from build123d import *

# Parameters (mm, degrees)
SKETCH_1_W      = 100
SKETCH_1_H      = 52
SKETCH_1_R      = 1.6
EXTRUDE_1_DEPTH = 3
FILLET_1_R      = 2


with BuildPart() as part:
    # 草图1 → 凸台-拉伸1 (new body)
    with BuildSketch(Plane(origin=(0, 0, 0), x_dir=(1, 0, 0), z_dir=(0, 1, 0))):
        Rectangle(SKETCH_1_W, SKETCH_1_H)
        with Locations(Location((-36.5, 17, 0), (0, 0, 270))):
            Circle(SKETCH_1_R, mode=Mode.SUBTRACT)
        with Locations(Location((36.5, 17, 0), (0, 0, 270))):
            Circle(SKETCH_1_R, mode=Mode.SUBTRACT)
        with Locations(Location((36.5, -19, 0), (0, 0, 270))):
            Circle(SKETCH_1_R, mode=Mode.SUBTRACT)
        with Locations(Location((-36.5, -19, 0), (0, 0, 270))):
            Circle(SKETCH_1_R, mode=Mode.SUBTRACT)
        with Locations(Location((-45, 19, 0), (0, 0, 270))):
            Circle(SKETCH_1_R, mode=Mode.SUBTRACT)
        with Locations(Location((45, 19, 0), (0, 0, 90))):
            Circle(SKETCH_1_R, mode=Mode.SUBTRACT)
        with Locations(Location((-45, -13, 0), (0, 0, 270))):
            Circle(SKETCH_1_R, mode=Mode.SUBTRACT)
        with Locations(Location((45, -13, 0), (0, 0, 90))):
            Circle(SKETCH_1_R, mode=Mode.SUBTRACT)
        with BuildLine():
            Line((-13, 0), (13, 0))
            ThreePointArc((13, 0), (14.414213562, 0.585786438), (15, 2))
            Line((15, 2), (15, 14))
            ThreePointArc((15, 14), (14.414213562, 15.414213562), (13, 16))
            Line((13, 16), (-13, 16))
            ThreePointArc((-13, 16), (-14.414213562, 15.414213562), (-15, 14))
            Line((-15, 14), (-15, 2))
            ThreePointArc((-15, 2), (-14.414213562, 0.585786438), (-13, 0))
        make_face(mode=Mode.SUBTRACT)
    extrude(amount=EXTRUDE_1_DEPTH)

    # 圆角1
    fillet_1_edges = [part.edges().sort_by_distance(p)[0] for p in [
        (50, 1.5, 26),
        (-50, 1.5, 26),
        (-50, 1.5, -26),
        (50, 1.5, -26),
    ]]
    fillet(fillet_1_edges, radius=FILLET_1_R)


solid = part.part
The listing builds one solid part. Answer for the finished solid, in the listing's coordinates (mm). A direction names the side the tool comes from. Give positions to 0.01 mm unless a question says otherwise; leave off trailing zeros. Loops run counter-clockwise (first coordinate to the right, second up) from the corner with the lowest first, then second, coordinate; pieces in that order, holes last. Notation, with made-up numbers: M 63,-28 L 86,-28 A25 ccw 86,4 Z; hole C 30.5,-7.5 d6. An arc over 180 degrees is marked long. Answer as CSV lines item,"result".
Item 1: The mould has two halves that part along X. Classify faces 3 (the flat face through (15, 1, -8)), 4 (the flat face through (50, 1, 0)), 5 (the flat face through (-1, 1, -26)), 6 (the cylindrical face through (35.53, 1.48, -18.27)): released by +X, released by -X, zero draft, split by the parting line, or undercut.
Values follow:
face 3,"undercut"
face 4,"released by +X"
face 5,"zero draft"
face 6,"undercut"
Item 2: The part is cut by section B-B (x = -3). Give the vertices of the cut face in (y, z).
Values follow:
outline,"M 0,-26 L 3,-26 L 3,-16 L 0,-16 Z; M 0,0 L 3,0 L 3,26 L 0,26 Z"
Item 3: The part is cut by section A-A (z = 13). Give the vertices of the cut face in (x, y), and give its area (3 significant figures).
Values follow:
outline,"M -50,0 L -46.6,0 L -46.6,3 L -50,3 Z; M -43.4,0 L 43.4,0 L 43.4,3 L -43.4,3 Z; M 46.6,0 L 50,0 L 50,3 L 46.6,3 Z"
area,"281 mm^2"
Item 4: Straight lines are drawn through the part: line 1 along X through (y, z) = (2.3, -19); line 2 along X through (y, z) = (2.25, 19); line 3 along Z through (x, y) = (45, 1.9). For each, find the intervals that lie inside material, in ascending order. Write a range as [from, to].
Values follow:
line 1,"x = [-50, -46.6], [-43.4, 43.4], [46.6, 50]"
line 2,"x = [-50, -38.1], [-34.9, 34.9], [38.1, 50]"
line 3,"z = [-26, -20.6], [-17.4, 11.4], [14.6, 26]"
Item 5: The part is cut by section D-D (y = 1.95). Give the number of separate pieces and of enclosed holes in the cut face, and give its area (3 significant figures).
Values follow:
separate pieces,"1"
enclosed holes,"9"
area,"4,660 mm^2"
Item 6: Given pin 1 Ø5 at (x, z) = (-45, -19) entering from +Y, flat-ended and moving along its own axis, determine where the tip first touches the part or whether it passes through.
Values follow:
pin 1,"stops at y = 3"
Item 7: Which of the six approach directions +Z, -Z, +X, -X, +Y, -Y give full straight-line access (tool end or side, diameter ignored) to faces 1 (the cylindrical face through (-49.43, 1.52, 25.4)), 2 (the cylindrical face through (-14.4, 1.48, -15.43))?
Values follow:
face 1,"+Z, -X, +Y, -Y"
face 2,"+Y, -Y"
Item 8: The part is cut by section C-C (z = -5). Give the vertices of the cut face in (x, y).
Values follow:
outline,"M -50,0 L -15,0 L -15,3 L -50,3 Z; M 15,0 L 50,0 L 50,3 L 15,3 Z"
